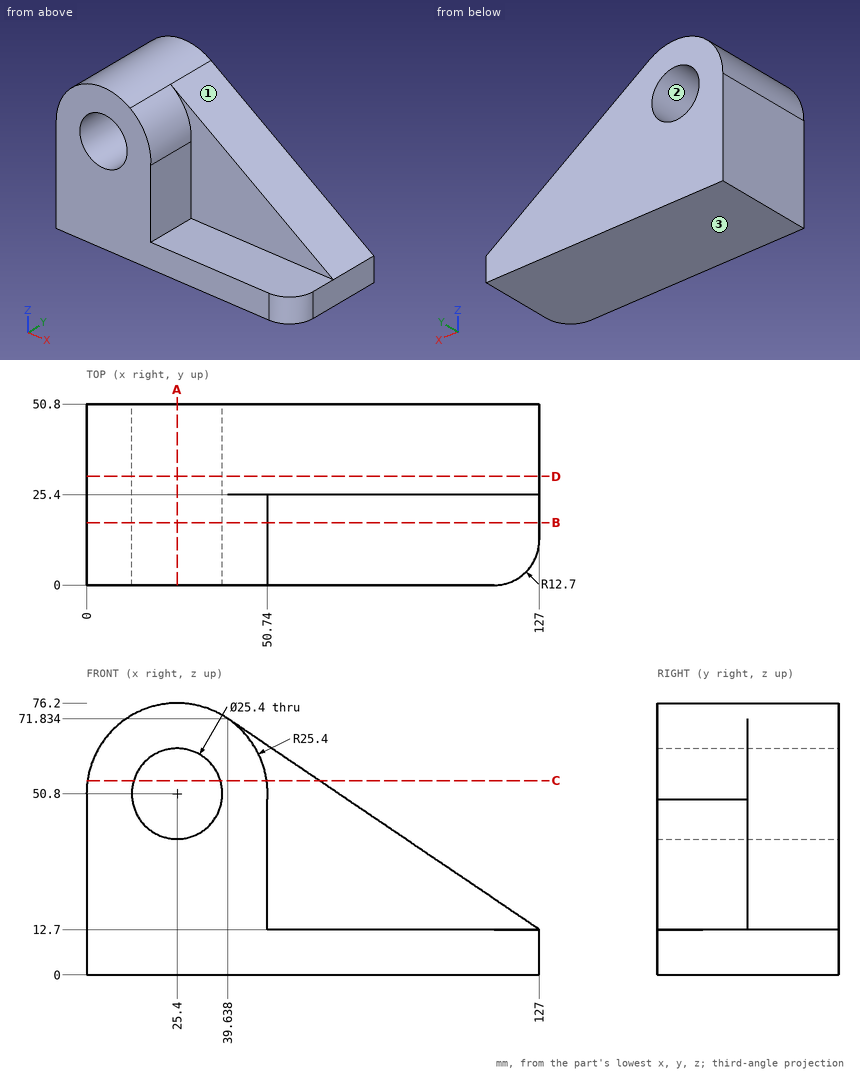
Here's the drawing with two shaded views (mm, measured from the low corner). I have some questions. Round coordinates to 2 decimals unless told otherwise and drop trailing zeros. Loops run counter-clockwise (first coordinate to the right, second up) from the corner with the lowest first, then second, coordinate; pieces in that order, holes last.
Item 1: Suppose I cut it at C-C, the plane z = 54.5. Write out the boundary of the cut face in (x, y), then the cut area to 3 significant figures.
Item 2: Suppose I cut it at D-D, the plane y = 30.5. Write out the boundary of the cut face in (x, z), then the cut area to 3 significant figures.
Item 3: Please list where these lines run through material, in increasing order: L1, parallel to X at y = 20, z = 50 (1 decimal); L2, parallel to Z at x = 25.4, y = 27.5; L3, parallel to Z at x = 102, y = 2.
Item 4: If we mould it in two halves opening along Z, with no side actions, what happens to the marked faces 1, 2 and 3? For each: +Z half, -Z half, draft (parallel to the pull), parting line (faces both ways), or undercut.
Item 5: Will these pins go through, and if not, where does the flat tip stop? pin 1 Ø1.5 at (x, y) = (53, 30.5) entering from +Z; pin 2 Ø7.5 at (x, y) = (73.5, 9) entering from +Z; pin 3 Ø7.5 at (y, z) = (9, 38) entering from +X; pin 4 Ø20.5 at (x, z) = (25.4, 50.8) entering from +Y.
Item 6: Suppose I cut it at B-B, the plane y = 17.5. Write out the boundary of the cut face in (x, z).
Item 7: Suppose I cut it at A-A, the plane x = 25.4. Write out the boundary of the cut face in (y, z), then the cut area to 3 significant figures.
Reported:
1. outline: (0.27, 0) - (13.25, 0) - (13.25, 50.8) - (0.27, 50.8) - close; (37.55, 0) - (50.53, 0) - (50.53, 25.4) - (65.25, 25.4) - (65.25, 50.8) - (37.55, 50.8) - close
1. area: 1,690 mm2
2. outline: (0, 0) - (127, 0) - (127, 12.7) - (39.64, 71.83) arc R25.4 ccw to (0, 50.8) - close; hole circle Ø25.4 at (25.4, 50.8)
2. area: 6,050 mm2
3. L1: x = 0 to 12.7, 38.1 to 50.8
3. L2: z = 0 to 38.1, 63.5 to 76.2
3. L3: z = 0 to 12.7
4. face 1: +Z half
4. face 2: undercut
4. face 3: -Z half
5. pin 1: stops at z = 63.3
5. pin 2: stops at z = 12.7
5. pin 3: stops at x = 50.74
5. pin 4: passes through
6. outline: (0, 0) - (127, 0) - (127, 12.7) - (50.74, 12.7) - (50.74, 49.06) arc R25.4 ccw (long way) to (0, 50.8) - close; hole circle Ø25.4 at (25.4, 50.8)
7. outline: (0, 0) - (50.8, 0) - (50.8, 38.1) - (0, 38.1) - close; (0, 63.5) - (50.8, 63.5) - (50.8, 76.2) - (0, 76.2) - close
7. area: 2,580 mm2
